```python
from build123d import *

# Parameters (mm, degrees)
SKETCH2_W          = 6
SKETCH2_H          = 0.5
CUT_EXTRUDE1_DEPTH = 6


with BuildPart() as part:
    # Sketch1 → Revolve1 (revolve)
    with BuildSketch(Plane.XY):
        Polygon((-5.8, 3), (-0.2, 3), (0, 3.2), (0, 4.5), (-1, 4.5), (-1, 5), (-6, 3.660254038), (-6, 3.2), align=None)
    revolve(axis=Axis((0, 0, 0), (-1, 0, 0)))

    # Sketch2 → Cut-Extrude1 (cut, through all)
    with BuildSketch(Plane(origin=(0, 0, 0), x_dir=(1, 0, 0), z_dir=(0, 1, 0))):
        with Locations((-3, 0)):
            Rectangle(SKETCH2_W, SKETCH2_H)
    extrude(amount=CUT_EXTRUDE1_DEPTH, mode=Mode.SUBTRACT)


solid = part.part
```
Part model, mm, in its own coordinate system. A direction names the side the tool comes from. Round coordinates to 2 decimals unless told otherwise and drop trailing zeros. Write each loop counter-clockwise with the first axis right and the second up, starting at its lowest first coordinate (ties: lowest second). Pieces come first, ordered by that corner, then holes. Notation, with made-up numbers: M -34.75,88.5 L -8.75,88.5 A19 cw -8.75,92.5 Z; hole C 69.5,-5.75 d10. An arc over 180 degrees is marked long. Answer as CSV lines item,"result". Start each with the question number.
1) Band-saw the part on D-D (x = -1.25). List the corners of the cut face in (y, z), then the cut area to 3 significant figures.
2) Band-saw the part on C-C (x = -3.3). List the corners of the cut face in (y, z), then the cut area to 3 significant figures.
3) Which spindle directions (+Z, -Z, +X, -X, +Y, -Y) get a long thin tool onto all of the face, cutting with end or side? Do faces 1 (the face through (-0.507, -4.496, -0.194)), 2 (the face through (0, -3, 2)), 3 (the face through (-2, 4, 0.25)). Say none if no direction does.
4) Band-saw the part on B-B (y = 0). List the corners of the cut face in (x, z), then the cut area to 3 significant figures.
5) Mould opens along Y. For faces 4 (the face through (-4.65, -4.02, -0.17)), 5 (the face through (-2, 4, -0.25)), 6 (the face through (-3, -3, 0)) say: +Y half, -Y half, draft (parallel to the pull), parting line (faces both ways), or undercut.
6) Drill centre lines: L1, parallel to Y at x = -1.6, z = 0.5; L2, parallel to Y at x = -0.4, z = -0.75; L3, parallel to Z at x = -4.5, y = 0.25. Where is each one in solid material? Low to high.
7) Band-saw the part on A-A (z = 0). List the corners of the cut face in (x, y), then the cut area to 3 significant figures.
8) Drop flat-ended pins along their axis: pin 1 (3 mm diameter, centred on x = -5, y = -2, fed in from +Z); pin 2 (1 mm diameter, centred on x = -3.5, y = 4, fed in from +Z); pin 3 (1.6 mm diameter, centred on x = -4, y = 4.5, fed in from -Z). Give the stop position or say it passes through.
Worked out:
1,outline,"M 2.99,-0.25 A3 cw long 2.99,0.25 L 4.93,0.25 A4.93 ccw long 4.93,-0.25 Z"
1,area,"47.2 mm²"
2,outline,"M 2.99,-0.25 A3 cw long 2.99,0.25 L 4.38,0.25 A4.38 ccw long 4.38,-0.25 Z"
2,area,"31.4 mm²"
3,face 1,"+X"
3,face 2,"+Z, -Z, +X, +Y, -Y"
3,face 3,"+X, -X, +Y"
4,outline,"M -6,-3.66 L -1,-5 L -1,-4.5 L 0,-4.5 L 0,-3.2 L -0.2,-3 L -5.8,-3 L -6,-3.2 Z; M -6,3.2 L -5.8,3 L -0.2,3 L 0,3.2 L 0,4.5 L -1,4.5 L -1,5 L -6,3.66 Z"
4,area,"16.2 mm²"
5,face 4,"parting line"
5,face 5,"draft"
5,face 6,"undercut"
6,L1,"-4.81 to -2.96, 2.96 to 4.81"
6,L2,"-4.44 to -2.9, 2.9 to 4.44"
6,L3,"-4.05 to -2.99, 2.99 to 4.05"
7,outline,"M -6,-3.66 L -1,-5 L -1,-4.5 L 0,-4.5 L 0,-3.2 L -0.2,-3 L -5.8,-3 L -6,-3.2 Z"
7,area,"8.11 mm²"
8,pin 1,"z = 4.11"
8,pin 2,"z = 2.59"
8,pin 3,"z = -2.05"
